Geometry: final body of the model. Coordinates: model frame, mm. Round coordinates to 2 decimals unless told otherwise and drop trailing zeros. Write each loop counter-clockwise with the first axis right and the second up, starting at its lowest first coordinate (ties: lowest second). Pieces come first, ordered by that corner, then holes. Notation, with made-up numbers: (55.5, 53) - (104.5, 53) arc R28 ccw to (104.5, 84) - close; hole circle Ø3 at (40, -26). An arc over 180 degrees is marked (long way). Use a Markdown table: item, result. Add a question column.
```python
from build123d import *

# Parameters (mm, degrees)
F1_DEPTH     = 177.8
F4_R         = 12.69999
F5_T1_DEPTH  = 6.4984e-06
F5_T3_DEPTH  = 6.4984e-06
F5_T5_DEPTH  = 6.4984e-06
F5_T7_DEPTH  = 6.4984e-06
F5_T9_DEPTH  = 6.4984e-06
F5_T11_DEPTH = 6.4984e-06
F5_T13_DEPTH = 6.4984e-06
F5_T15_DEPTH = 6.4984e-06
F5_T17_DEPTH = 6.4984e-06
F5_T20_ANGLE = 36
F5_T22_ANGLE = 36
F5_T24_ANGLE = 36
F5_T26_ANGLE = 36
F5_T28_ANGLE = 36
F5_T30_ANGLE = 36
F5_T32_ANGLE = 36
F5_T34_ANGLE = 36
F5_T36_ANGLE = 36
F5_T38_ANGLE = 36


# Not quite as in the source:
# - a fillet or chamfer that OpenCascade refuses, or shapes differently, is made with other operations: its cross-section is extruded or revolved along the edge and cut away or added
# - a fillet or chamfer is up to 0.001 mm smaller than in the source, because OpenCascade refuses the exact size


with BuildPart() as f1:
    # F0 (on Top) → F1 (new body)
    with BuildSketch(Plane.XY):
        Polygon((-12.7, 4.1264801422), (-12.7, -4.1264801422), (-7.8490316571, -10.8032652661), (0, -13.3535702478), (7.8490316571, -10.8032652661), (12.7, -4.1264801422), (12.7, 4.1264801422), (7.8490316571, 10.8032652661), (0, 13.3535702478), (-7.8490316571, 10.8032652661), align=None)
    extrude(amount=F1_DEPTH)

    # F1_face (on face) → F3 section 0
    with BuildSketch(Plane.XY.offset(177.8), mode=Mode.PRIVATE) as f3_s0:
        Polygon((-7.8490316571, 10.8032652661), (-12.7, 4.1264801422), (-12.7, -4.1264801422), (-7.8490316571, -10.8032652661), (0, -13.3535702478), (7.8490316571, -10.8032652661), (12.7, -4.1264801422), (12.7, 4.1264801422), (7.8490316571, 10.8032652661), (0, 13.3535702478), align=None)
    loft([f3_s0.sketch, Vertex(0, 0, 201.3573497534)])

    # F4 (radius 12.7 in the source; OpenCascade refuses exactly that, so slightly less here)
    f4_edges = [f1.edges().sort_by_distance(p)[0] for p in [
        (0, -13.35357, 88.9),
        (-7.849032, -10.803265, 88.9),
        (-12.7, -4.12648, 88.9),
        (-12.7, 4.12648, 88.9),
        (-7.849032, 10.803265, 88.9),
        (0, 13.35357, 88.9),
        (7.849032, 10.803265, 88.9),
        (12.7, 4.12648, 88.9),
        (12.7, -4.12648, 88.9),
        (7.849032, -10.803265, 88.9),
    ]]
    fillet(f4_edges, radius=F4_R)

    # F5: fillet of radius 5.08 on 1 edges, made by hand

    # F5_s2 → F5_t1 (cut)
    with BuildSketch(Plane.XZ.offset(-3.2492e-06)):
        with BuildLine():
            ThreePointArc((-7.62, 0), (-11.2121024484, 1.4878975516), (-12.7, 5.08))
            Line((-12.7, 5.08), (-12.7, 0))
            Line((-12.7, 0), (-7.62, 0))
        make_face()
        with BuildLine():
            ThreePointArc((7.62, 0), (11.2121024484, 1.4878975516), (12.7, 5.08))
            Line((12.7, 5.08), (12.7, 0))
            Line((12.7, 0), (7.62, 0))
        make_face()
    extrude(amount=F5_T1_DEPTH, mode=Mode.SUBTRACT)

    # F5_s4 → F5_t3 (cut)
    with BuildSketch(Plane(origin=(-1.9098e-06, 2.6287e-06, 0), x_dir=(0, 0, 1), z_dir=(0.5877852523, -0.8090169944, 0))):
        with BuildLine():
            ThreePointArc((0, 7.62), (1.4878975516, 11.2121024484), (5.08, 12.7))
            Line((5.08, 12.7), (0, 12.7))
            Line((0, 12.7), (0, 7.62))
        make_face()
    extrude(amount=F5_T3_DEPTH, mode=Mode.SUBTRACT)

    # F5_s6 → F5_t5 (cut)
    with BuildSketch(Plane(origin=(-3.0902e-06, 1.0041e-06, 0), x_dir=(0, 0, 1), z_dir=(0.9510565163, -0.3090169944, 0))):
        with BuildLine():
            ThreePointArc((0, 7.62), (1.4878975516, 11.2121024484), (5.08, 12.7))
            Line((5.08, 12.7), (0, 12.7))
            Line((0, 12.7), (0, 7.62))
        make_face()
    extrude(amount=F5_T5_DEPTH, mode=Mode.SUBTRACT)

    # F5_s8 → F5_t7 (cut)
    with BuildSketch(Plane(origin=(-3.0902e-06, -1.0041e-06, 0), x_dir=(0, 0, 1), z_dir=(0.9510565163, 0.3090169944, 0))):
        with BuildLine():
            ThreePointArc((0, 7.62), (1.4878975516, 11.2121024484), (5.08, 12.7))
            Line((5.08, 12.7), (0, 12.7))
            Line((0, 12.7), (0, 7.62))
        make_face()
    extrude(amount=F5_T7_DEPTH, mode=Mode.SUBTRACT)

    # F5_s10 → F5_t9 (cut)
    with BuildSketch(Plane(origin=(-1.9098e-06, -2.6287e-06, 0), x_dir=(0, 0, 1), z_dir=(0.5877852523, 0.8090169944, 0))):
        with BuildLine():
            ThreePointArc((0, 7.62), (1.4878975516, 11.2121024484), (5.08, 12.7))
            Line((5.08, 12.7), (0, 12.7))
            Line((0, 12.7), (0, 7.62))
        make_face()
    extrude(amount=F5_T9_DEPTH, mode=Mode.SUBTRACT)

    # F5_s12 → F5_t11 (cut)
    with BuildSketch(Plane(origin=(1.9098e-06, -2.6287e-06, 0), x_dir=(0, 0, 1), z_dir=(-0.5877852523, 0.8090169944, 0))):
        with BuildLine():
            ThreePointArc((0, 7.62), (1.4878975516, 11.2121024484), (5.08, 12.7))
            Line((5.08, 12.7), (0, 12.7))
            Line((0, 12.7), (0, 7.62))
        make_face()
    extrude(amount=F5_T11_DEPTH, mode=Mode.SUBTRACT)

    # F5_s14 → F5_t13 (cut)
    with BuildSketch(Plane(origin=(3.0902e-06, -1.0041e-06, 0), x_dir=(0, 0, 1), z_dir=(-0.9510565163, 0.3090169944, 0))):
        with BuildLine():
            ThreePointArc((0, 7.62), (1.4878975516, 11.2121024484), (5.08, 12.7))
            Line((5.08, 12.7), (0, 12.7))
            Line((0, 12.7), (0, 7.62))
        make_face()
    extrude(amount=F5_T13_DEPTH, mode=Mode.SUBTRACT)

    # F5_s16 → F5_t15 (cut)
    with BuildSketch(Plane(origin=(3.0902e-06, 1.0041e-06, 0), x_dir=(0, 0, 1), z_dir=(-0.9510565163, -0.3090169944, 0))):
        with BuildLine():
            ThreePointArc((0, 7.62), (1.4878975516, 11.2121024484), (5.08, 12.7))
            Line((5.08, 12.7), (0, 12.7))
            Line((0, 12.7), (0, 7.62))
        make_face()
    extrude(amount=F5_T15_DEPTH, mode=Mode.SUBTRACT)

    # F5_s18 → F5_t17 (cut)
    with BuildSketch(Plane(origin=(1.9098e-06, 2.6287e-06, 0), x_dir=(0, 0, 1), z_dir=(-0.5877852523, -0.8090169944, 0))):
        with BuildLine():
            ThreePointArc((5.08, 12.7), (1.4878975516, 11.2121024484), (0, 7.62))
            Line((0, 7.62), (0, 12.7))
            Line((0, 12.7), (5.08, 12.7))
        make_face()
    extrude(amount=F5_T17_DEPTH, mode=Mode.SUBTRACT)

    # F5_s19 → F5_t20 (revolve, cut)
    with BuildSketch(Plane.XZ.offset(3.2492e-06)):
        with BuildLine():
            ThreePointArc((-7.62, 0), (-11.2121024484, 1.4878975516), (-12.7, 5.08))
            Line((-12.7, 5.08), (-12.7, 0))
            Line((-12.7, 0), (-7.62, 0))
        make_face()
    revolve(axis=Axis((-1e-05, -3.2492e-06, 0), (0, 0, 1)), revolution_arc=F5_T20_ANGLE, mode=Mode.SUBTRACT)

    # F5_s21 → F5_t22 (revolve, cut)
    with BuildSketch(Plane(origin=(1.9098e-06, -2.6287e-06, 0), x_dir=(0, 0, 1), z_dir=(-0.5877852523, 0.8090169944, 0))):
        with BuildLine():
            ThreePointArc((0, -7.62), (1.4878975516, -11.2121024484), (5.08, -12.7))
            Line((5.08, -12.7), (0, -12.7))
            Line((0, -12.7), (0, -7.62))
        make_face()
    revolve(axis=Axis((-6.1803e-06, -8.5065e-06, 0), (0, 0, 1)), revolution_arc=F5_T22_ANGLE, mode=Mode.SUBTRACT)

    # F5_s23 → F5_t24 (revolve, cut)
    with BuildSketch(Plane(origin=(3.0902e-06, -1.0041e-06, 0), x_dir=(0, 0, 1), z_dir=(-0.9510565163, 0.3090169944, 0))):
        with BuildLine():
            ThreePointArc((0, -7.62), (1.4878975516, -11.2121024484), (5.08, -12.7))
            Line((5.08, -12.7), (0, -12.7))
            Line((0, -12.7), (0, -7.62))
        make_face()
    revolve(axis=Axis((0, -1.05146e-05, 0), (0, 0, 1)), revolution_arc=F5_T24_ANGLE, mode=Mode.SUBTRACT)

    # F5_s25 → F5_t26 (revolve, cut)
    with BuildSketch(Plane(origin=(3.0902e-06, 1.0041e-06, 0), x_dir=(0, 0, 1), z_dir=(-0.9510565163, -0.3090169944, 0))):
        with BuildLine():
            ThreePointArc((0, -7.62), (1.4878975516, -11.2121024484), (5.08, -12.7))
            Line((5.08, -12.7), (0, -12.7))
            Line((0, -12.7), (0, -7.62))
        make_face()
    revolve(axis=Axis((6.1803e-06, -8.5065e-06, 0), (0, 0, 1)), revolution_arc=F5_T26_ANGLE, mode=Mode.SUBTRACT)

    # F5_s27 → F5_t28 (revolve, cut)
    with BuildSketch(Plane(origin=(1.9098e-06, 2.6287e-06, 0), x_dir=(0, 0, 1), z_dir=(-0.5877852523, -0.8090169944, 0))):
        with BuildLine():
            ThreePointArc((0, -7.62), (1.4878975516, -11.2121024484), (5.08, -12.7))
            Line((5.08, -12.7), (0, -12.7))
            Line((0, -12.7), (0, -7.62))
        make_face()
    revolve(axis=Axis((1e-05, -3.2492e-06, 0), (0, 0, 1)), revolution_arc=F5_T28_ANGLE, mode=Mode.SUBTRACT)

    # F5_s29 → F5_t30 (revolve, cut)
    with BuildSketch(Plane.XZ.offset(-3.2492e-06)):
        with BuildLine():
            ThreePointArc((7.62, 0), (11.2121024484, 1.4878975516), (12.7, 5.08))
            Line((12.7, 5.08), (12.7, 0))
            Line((12.7, 0), (7.62, 0))
        make_face()
    revolve(axis=Axis((1e-05, 3.2492e-06, 0), (0, 0, 1)), revolution_arc=F5_T30_ANGLE, mode=Mode.SUBTRACT)

    # F5_s31 → F5_t32 (revolve, cut)
    with BuildSketch(Plane(origin=(3.0902e-06, -1.0041e-06, 0), x_dir=(0, 0, 1), z_dir=(-0.9510565163, 0.3090169944, 0))):
        with BuildLine():
            ThreePointArc((0, 7.62), (1.4878975516, 11.2121024484), (5.08, 12.7))
            Line((5.08, 12.7), (0, 12.7))
            Line((0, 12.7), (0, 7.62))
        make_face()
    revolve(axis=Axis((6.1803e-06, 8.5065e-06, 0), (0, 0, -1)), revolution_arc=F5_T32_ANGLE, mode=Mode.SUBTRACT)

    # F5_s33 → F5_t34 (revolve, cut)
    with BuildSketch(Plane(origin=(3.0902e-06, 1.0041e-06, 0), x_dir=(0, 0, 1), z_dir=(-0.9510565163, -0.3090169944, 0))):
        with BuildLine():
            ThreePointArc((0, 7.62), (1.4878975516, 11.2121024484), (5.08, 12.7))
            Line((5.08, 12.7), (0, 12.7))
            Line((0, 12.7), (0, 7.62))
        make_face()
    revolve(axis=Axis((0, 1.05146e-05, 0), (0, 0, -1)), revolution_arc=F5_T34_ANGLE, mode=Mode.SUBTRACT)

    # F5_s35 → F5_t36 (revolve, cut)
    with BuildSketch(Plane(origin=(1.9098e-06, 2.6287e-06, 0), x_dir=(0, 0, 1), z_dir=(-0.5877852523, -0.8090169944, 0))):
        with BuildLine():
            ThreePointArc((0, 7.62), (1.4878975516, 11.2121024484), (5.08, 12.7))
            Line((5.08, 12.7), (0, 12.7))
            Line((0, 12.7), (0, 7.62))
        make_face()
    revolve(axis=Axis((-6.1803e-06, 8.5065e-06, 0), (0, 0, -1)), revolution_arc=F5_T36_ANGLE, mode=Mode.SUBTRACT)

    # F5_s37 → F5_t38 (revolve, cut)
    with BuildSketch(Plane(origin=(-1.9098e-06, -2.6287e-06, 0), x_dir=(0, 0, 1), z_dir=(0.5877852523, 0.8090169944, 0))):
        with BuildLine():
            ThreePointArc((0, -7.62), (1.4878975516, -11.2121024484), (5.08, -12.7))
            Line((5.08, -12.7), (0, -12.7))
            Line((0, -12.7), (0, -7.62))
        make_face()
    revolve(axis=Axis((-1e-05, 3.2492e-06, 0), (0, 0, 1)), revolution_arc=F5_T38_ANGLE, mode=Mode.SUBTRACT)


solid = f1.part
```
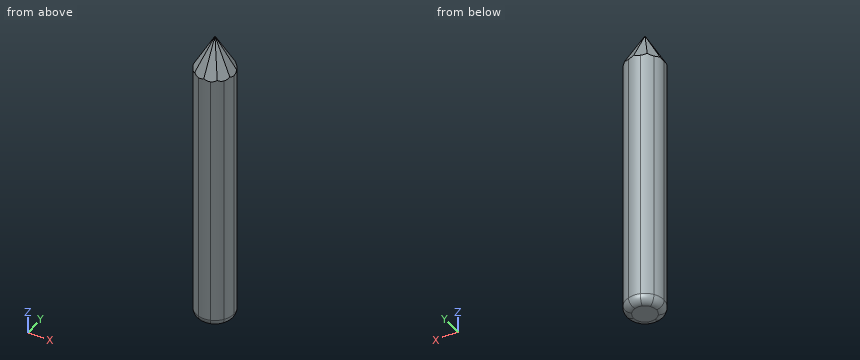
1) Pin query (flat end, axial travel): P1, Ø3, axis at x = -7.5, y = -7.5, coming from the -Z side; P2, Ø6, axis at x = 4, y = -3.5, coming from the +Z side; P3, Ø1, axis at y = -2, z = 63, coming from the -X side. Return the tip coordinate at first contact, or that it passes through.
2) Section B-B, the plane z = 184.5. Return the cut outline in (x, y), then the cut area to 3 significant figures.
3) Material intervals for L1, parallel to X at y = -7.5, z = 116; L2, parallel to X at y = -0.5, z = 22.5, sorted ascending. Write a range as from..to.
Output values:
| question | item | result |
|---|---|---|
| 1 | P1 | stops at z = 0.22 |
| 1 | P2 | stops at z = 197.1 |
| 1 | P3 | stops at x = -12.61 |
| 2 | outline | (-9.09, -2.95) - (-5.62, -7.73) - (0, -9.56) - (5.62, -7.73) - (9.09, -2.95) - (9.09, 2.95) - (5.62, 7.73) - (0, 9.56) - (-5.62, 7.73) - (-9.09, 2.95) - close |
| 2 | area | 268 mm^2 |
| 3 | L1 | x = -10.25..10.25 |
| 3 | L2 | x = -12.69..12.69 |
